```python
from build123d import *

# Parameters (mm, degrees)
F0_W     = 60
F0_H     = 40
F0_W_2   = 54
F0_H_2   = 34
F1_DEPTH = 600
F2_R     = 30
F3_DEPTH = 60
F4_DEPTH = 25


with BuildPart() as f1:
    # F0 (on Right) → F1 (new body)
    with BuildSketch(Plane.YZ):
        with Locations((-30, -0.412365)):
            Rectangle(F0_W, F0_H)
        with Locations((-30, -0.412365)):
            Rectangle(F0_W_2, F0_H_2, mode=Mode.SUBTRACT)
    extrude(amount=F1_DEPTH)

    # F2 (on face) → F3 (cut)
    with BuildSketch(Plane(origin=(0, 0, 0), x_dir=(-1, 0, 0), z_dir=(0, 1, 0))):
        with BuildLine():
            ThreePointArc((-586.55, -13.862365), (-577.039414, -9.922951), (-573.1, -0.412365))
            ThreePointArc((-573.1, -0.412365), (-577.039414, 9.098221), (-586.55, 13.037635))
            ThreePointArc((-586.55, 13.037635), (-600, -0.412365), (-586.55, -13.862365))
        make_face()
        Circle(F2_R)
        with BuildLine():
            ThreePointArc((-600, -0.412365), (-596.060586, 9.098221), (-586.55, 13.037635))
            Line((-586.55, 13.037635), (-600, 13.037635))
            Line((-600, 13.037635), (-600, -0.412365))
        make_face()
        with BuildLine():
            Line((-600, -13.862365), (-586.55, -13.862365))
            ThreePointArc((-586.55, -13.862365), (-596.060586, -9.922951), (-600, -0.412365))
            Line((-600, -0.412365), (-600, -13.862365))
        make_face()
    extrude(amount=-F3_DEPTH, mode=Mode.SUBTRACT)

    # F2 (on face) → F4 (cut)
    with BuildSketch(Plane(origin=(0, 0, 0), x_dir=(-1, 0, 0), z_dir=(0, 1, 0))):
        with BuildLine():
            ThreePointArc((-586.55, -13.862365), (-577.039414, -9.922951), (-573.1, -0.412365))
            ThreePointArc((-573.1, -0.412365), (-577.039414, 9.098221), (-586.55, 13.037635))
            ThreePointArc((-586.55, 13.037635), (-600, -0.412365), (-586.55, -13.862365))
        make_face()
        Circle(F2_R)
    extrude(amount=-F4_DEPTH, mode=Mode.SUBTRACT)


solid = f1.part
```
Source: CAD feature listing. Evaluate the final solid. Frame: model axes, mm. A direction names the side the tool comes from. Give positions to 0.01 mm unless a question says otherwise; leave off trailing zeros. Order: outer loops, then holes, each group sorted by start corner. A loop starts at its lowest first (then second) coordinate and runs counter-clockwise, first axis right, second up.
(1) Section query B-B (x = 121). Return the cut outline in (y, z).
(2) Contact query for a flat-ended pin moving along its axis: P1, Ø12, axis at y = -35, z = -13.5, coming from the -X side. Output: stop coordinate, or through.
(3) Access query for faces 1 (the face through (308, -57, -1)), 2 (the face through (307, -60, -1)). Directions: +Z, -Z, +X, -X, +Y, -Y. A direction counts if a zero-diameter tool reaches every point of the face in a straight line with its end or side. Return the directions, or none.
(4) Section query A-A (y = -35.5). Return the cut outline in (x, z).
(5) Pull-direction query (Z, two-part tool) for faces 3 (the face through (308, -3, -1)), 4 (the face through (307, -30, -20.412)), 5 (the face through (307, -30, 19.588)), 6 (the face through (307, 0, -1)); classes: +Z half, -Z half, draft (parallel to the pull), parting line (faces both ways), or undercut.
(6) Material intervals for line 1 along Z through (x, y) = (433.5, -19.5); line 2 along Y through (x, z) = (341.5, 3), sorted ascending.
(7) Section query C-C (z = -7). Return the cut outline in (x, y).
Outcome:
1. outline: (-60, -20.41) - (0, -20.41) - (0, 19.59) - (-60, 19.59) - close; hole (-57, -17.41) - (-3, -17.41) - (-3, 16.59) - (-57, 16.59) - close
2. P1: stops at x = 22.8
3. face 1: +X, -X
3. face 2: +Z, -Z, +X, -X, -Y
4. outline: (21.98, -20.41) - (600, -20.41) - (600, -17.41) - (24.43, -17.41) arc R30 cw to start; (22.72, 19.59) arc R30 cw to (25, 16.59) - (600, 16.59) - (600, 19.59) - close
5. face 3: undercut
5. face 4: -Z half
5. face 5: +Z half
5. face 6: draft
6. line 1: z = -20.41 to -17.41, 16.59 to 19.59
6. line 2: y = -60 to -57, -3 to 0
7. outline: (29.17, -60) - (574.82, -60) - (574.82, -57) - (29.17, -57) - close; (29.17, -3) - (574.82, -3) - (574.82, 0) - (29.17, 0) - close
